Verification items for this drawing (mm, ordinates from the low corner). A direction names the side the tool comes from. Coordinates: 2 decimals unless noted, no trailing zeros. Order: outer loops, then holes, each group sorted by start corner. A loop starts at its lowest first (then second) coordinate and runs counter-clockwise, first axis right, second up. Notation, with made-up numbers: (5, 13) -> (51, 13) arc R28 cw to (51, 37) -> close; hole circle Ø9 at (27, 87.5). An arc over 180 degrees is marked (long way). Write item = value, one per line. Start each with the question number.
1. Go/stop test with flat-tipped pins: P1, Ø4.5, axis at x = 4, z = 5, coming from the -Y side; P2, Ø9, axis at x = 16.5, y = 16, coming from the -Z side; P3, Ø2.5, axis at x = 3.5, z = 8, coming from the +Y side. Record where each tip stops, or that it passes through.
2. Thickness scan on line 1 along Y through (x, z) = (17, 9.25); line 2 along X through (y, z) = (31.7, 11.2); line 3 along X through (y, z) = (17.7, 10.5). Record the ranges inside material, lowest first. Write a range as from..to.
3. Cross-section at A-A on z = 5. Give the number of separate pieces and of enclosed holes in the cut face, plus the area to 3 significant figures.
4. Set-up check for the marked faces 1, 2 and 3: record each of +Z, -Z, +X, -X, +Y, -Y from which the full face is reachable in a straight line by a thin tool's end or side.
5. Release check for a two-part mould opening along Y. For the marked faces 4, 5, 6 and 7 record: +Y half, -Y half, draft (parallel to the pull), parting line (faces both ways), or undercut.
6. Cross-section at D-D on z = 1.75. Record the cut outline in (x, y).
7. Cross-section at B-B on x = 70. Record the cut outline in (y, z).
8. Cross-section at C-C on y = 31.7. Record the cut outline in (x, z).
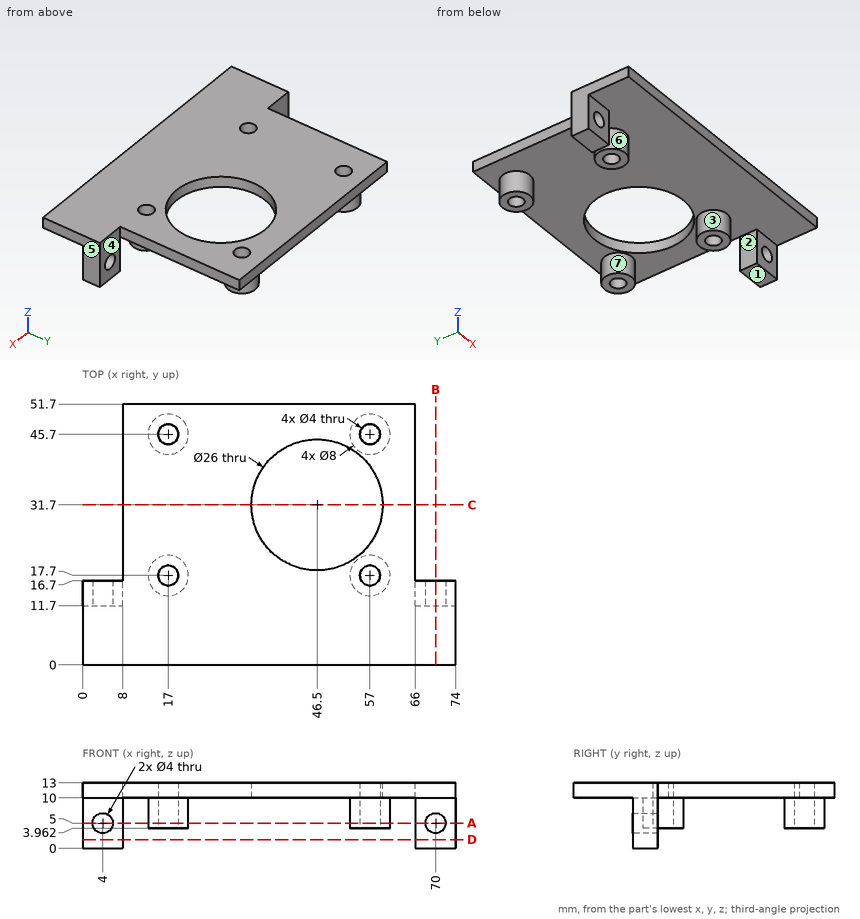
Worked out:
q1.P1 = 11.7
q1.P2 = 3.96
q1.P3 = 16.7
q2.line_1 = 13.7..15.7, 19.7..21.7, 41.7..43.7, 47.7..49.7
q2.line_2 = 8..33.5, 59.5..66
q2.line_3 = 8..15, 19..55, 59..66
q3.separate_pieces = 8
q3.enclosed_holes = 4
q3.area = 191 mm²
q4.face_1 = -Z, +X, -X, +Y, -Y
q4.face_2 = -Z, +Y, -Y
q4.face_3 = -Z
q5.face_4 = +Y half
q5.face_5 = draft
q5.face_6 = undercut
q5.face_7 = undercut
q6.outline = (0, 11.7) -> (8, 11.7) -> (8, 16.7) -> (0, 16.7) -> close; (66, 11.7) -> (74, 11.7) -> (74, 16.7) -> (66, 16.7) -> close
q7.outline = (0, 10) -> (11.7, 10) -> (11.7, 7) -> (16.7, 7) -> (16.7, 13) -> (0, 13) -> close; (11.7, 0) -> (16.7, 0) -> (16.7, 3) -> (11.7, 3) -> close
q8.outline = (8, 10) -> (33.5, 10) -> (33.5, 13) -> (8, 13) -> close; (59.5, 10) -> (66, 10) -> (66, 13) -> (59.5, 13) -> close
